```python
from build123d import *

# Parameters (mm, degrees)
SKETCH2_W           = 93
SKETCH2_H           = 50
BOSS_EXTRUDE1_DEPTH = 3
SKETCH1_R           = 1.5
SKETCH1_R_2         = 2
CUT_EXTRUDE9_DEPTH  = 4


with BuildPart() as part:
    # Sketch2 → Boss-Extrude1 (new body)
    with BuildSketch(Plane.XY):
        Rectangle(SKETCH2_W, SKETCH2_H)
    extrude(amount=BOSS_EXTRUDE1_DEPTH)

    # Sketch1 → Cut-Extrude9 (cut, through all)
    with BuildSketch(Plane.XY):
        with BuildLine():
            ThreePointArc((21.629165125, 3.25), (20.596194078, 4.596194078), (19.25, 5.629165125))
            Line((19.25, 5.629165125), (19.25, 18.5))
            Line((19.25, 18.5), (34.132524712, 18.5))
            ThreePointArc((34.132524712, 18.5), (36.249054116, 15.045959438), (40, 13.516090852))
            Line((40, 13.516090852), (40, 3.25))
            Line((40, 3.25), (21.629165125, 3.25))
        make_face()
        with BuildLine():
            ThreePointArc((12.75, 5.629165125), (11.403805922, 4.596194078), (10.370834875, 3.25))
            Line((10.370834875, 3.25), (-8.370834875, 3.25))
            ThreePointArc((-8.370834875, 3.25), (-9.403805922, 4.596194078), (-10.75, 5.629165125))
            Line((-10.75, 5.629165125), (-10.75, 18.5))
            Line((-10.75, 18.5), (12.75, 18.5))
            Line((12.75, 18.5), (12.75, 5.629165125))
        make_face()
        with BuildLine():
            ThreePointArc((-40, 13.67544468), (-36.903805922, 15.403805922), (-35.17544468, 18.5))
            Line((-35.17544468, 18.5), (-17.25, 18.5))
            Line((-17.25, 18.5), (-17.25, 5.629165125))
            ThreePointArc((-17.25, 5.629165125), (-18.596194078, 4.596194078), (-19.629165125, 3.25))
            Line((-19.629165125, 3.25), (-28.370834875, 3.25))
            ThreePointArc((-28.370834875, 3.25), (-34, 6.5), (-39.629165125, 3.25))
            Line((-39.629165125, 3.25), (-40, 3.25))
            Line((-40, 3.25), (-40, 13.67544468))
        make_face()
        with BuildLine():
            ThreePointArc((-35.871480673, -18.5), (-37.618576198, -16.537237855), (-40, -15.426562977))
            Line((-40, -15.426562977), (-40, -3.25))
            Line((-40, -3.25), (-39.629165125, -3.25))
            ThreePointArc((-39.629165125, -3.25), (-34, -6.5), (-28.370834875, -3.25))
            Line((-28.370834875, -3.25), (-19.629165125, -3.25))
            ThreePointArc((-19.629165125, -3.25), (-18.596194078, -4.596194078), (-17.25, -5.629165125))
            Line((-17.25, -5.629165125), (-17.25, -18.5))
            Line((-17.25, -18.5), (-35.871480673, -18.5))
        make_face()
        with BuildLine():
            ThreePointArc((-10.75, -5.629165125), (-9.403805922, -4.596194078), (-8.370834875, -3.25))
            Line((-8.370834875, -3.25), (10.370834875, -3.25))
            ThreePointArc((10.370834875, -3.25), (11.403805922, -4.596194078), (12.75, -5.629165125))
            Line((12.75, -5.629165125), (12.75, -18.5))
            Line((12.75, -18.5), (-10.75, -18.5))
            Line((-10.75, -18.5), (-10.75, -5.629165125))
        make_face()
        with BuildLine():
            ThreePointArc((19.25, -5.629165125), (20.596194078, -4.596194078), (21.629165125, -3.25))
            Line((21.629165125, -3.25), (40, -3.25))
            Line((40, -3.25), (40, -15.267209149))
            ThreePointArc((40, -15.267209149), (37.011595442, -16.239436527), (34.828560705, -18.5))
            Line((34.828560705, -18.5), (19.25, -18.5))
            Line((19.25, -18.5), (19.25, -5.629165125))
        make_face()
        with Locations((40.457080032, 20)):
            Circle(SKETCH1_R)
        with Locations((-41.5, 20)):
            Circle(SKETCH1_R)
        with Locations((-34, 0)):
            Circle(SKETCH1_R_2)
        with Locations((-14, 0)):
            Circle(SKETCH1_R_2)
        with Locations((16, 0)):
            Circle(SKETCH1_R_2)
        with Locations((40.457080032, -21.751118297)):
            Circle(SKETCH1_R)
        with Locations((-41.5, -21.751118297)):
            Circle(SKETCH1_R)
    extrude(amount=CUT_EXTRUDE9_DEPTH, mode=Mode.SUBTRACT)


solid = part.part
```
Check sheet for the modelled part. Datum: model origin and axes. Units: mm. Round coordinates to 2 decimals unless told otherwise and drop trailing zeros. Order: outer loops, then holes, each group sorted by start corner. A loop starts at its lowest first (then second) coordinate and runs counter-clockwise, first axis right, second up.
1) Section check B-B (y = 20). Record the boundary of the cut face in (x, z).
2) Mould release check, pull along X, two halves, no side actions. Record for faces 1 (the flat face through (-24, -3.25, 1)), 2 (the flat face through (46.5, 0, 1)): +X half, -X half, draft (parallel to the pull), parting line (faces both ways), or undercut.
3) Section check A-A (x = -7.5). Record the boundary of the cut face in (y, z), and give its area (3 significant figures).
4) Scan lines: line 1 (X direction, y = 20, z = 2); line 2 (Y direction, x = 23, z = 1.65); line 3 (Y direction, x = -41.5, z = 1.7). Record each from-to range of solid material in increasing order.
5) Go/stop test with flat-tipped pins: pin 1 Ø5 at (x, y) = (-41.5, 20) entering from -Z; pin 2 Ø3.5 at (x, y) = (-14, 0) entering from +Z. Record where each tip stops, or that it passes through.
6) Section check C-C (x = 16). Record the boundary of the cut face in (y, z).
7) Section check D-D (y = -11.5). Record the boundary of the cut face in (x, z).
Result:
1. outline: (-46.5, 0) - (-43, 0) - (-43, 3) - (-46.5, 3) - close; (-40, 0) - (38.96, 0) - (38.96, 3) - (-40, 3) - close; (41.96, 0) - (46.5, 0) - (46.5, 3) - (41.96, 3) - close
2. face 1: undercut
2. face 2: +X half
3. outline: (-25, 0) - (-18.5, 0) - (-18.5, 3) - (-25, 3) - close; (-3.25, 0) - (3.25, 0) - (3.25, 3) - (-3.25, 3) - close; (18.5, 0) - (25, 0) - (25, 3) - (18.5, 3) - close
3. area: 58.5 mm2
4. line 1: x = -46.5 to -43, -40 to 38.96, 41.96 to 46.5
4. line 2: y = -25 to -18.5, -3.25 to 3.25, 18.5 to 25
4. line 3: y = -25 to -23.25, -20.25 to 18.5, 21.5 to 25
5. pin 1: stops at z = 0
5. pin 2: passes through
6. outline: (-25, 0) - (-2, 0) - (-2, 3) - (-25, 3) - close; (2, 0) - (25, 0) - (25, 3) - (2, 3) - close
7. outline: (-46.5, 0) - (-40, 0) - (-40, 3) - (-46.5, 3) - close; (-17.25, 0) - (-10.75, 0) - (-10.75, 3) - (-17.25, 3) - close; (12.75, 0) - (19.25, 0) - (19.25, 3) - (12.75, 3) - close; (40, 0) - (46.5, 0) - (46.5, 3) - (40, 3) - close
